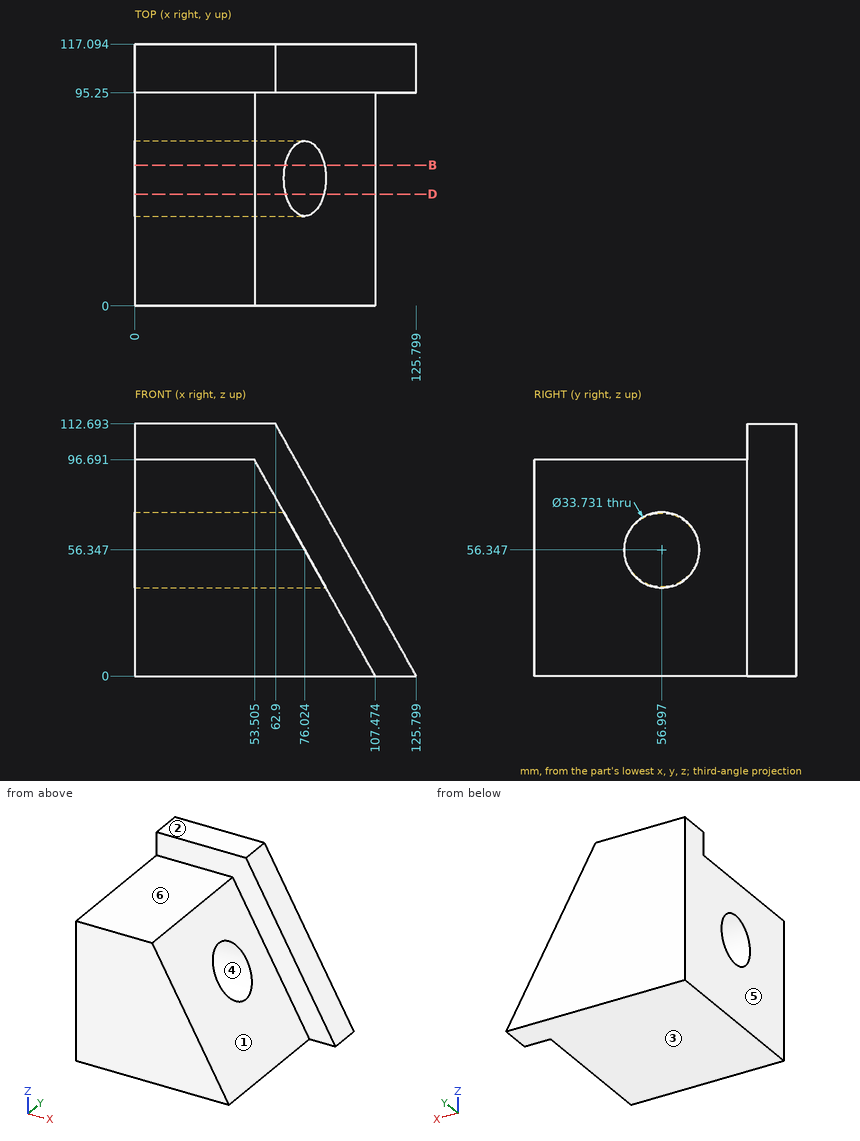
Part print with two shaded views. Sizes in mm from the minimum x, y, z corner. A direction names the side the tool comes from. Give positions to 0.01 mm unless a question says otherwise; leave off trailing zeros. Order: outer loops, then holes, each group sorted by start corner. A loop starts at its lowest first (then second) coordinate and runs counter-clockwise, first axis right, second up. Notation, with made-up numbers: (8, 78) - (66, 78) arc R19 ccw to (66, 104) - close; hole circle Ø2 at (9, 11.5). An arc over 180 degrees is marked (long way). Write each question's results on one line, items separated by ' | '.
1. Pull direction Z, two halves, no side cores. Call the marked faces 3, 4, 5 and 6: released by +Z, released by -Z, zero draft, split by the parting line, or undercut.
Calculated:
face 3: released by -Z | face 4: undercut | face 5: zero draft | face 6: released by +Z
2. 3-axis set-ups, long thin cutter, end or side, ignore diameter. For the marked faces 1 and 2: which of +Z, -Z, +X, -X, +Y, -Y reach the whole face in a straight line?
Calculated:
face 1: +Z, +X, -Y | face 2: +Z, +X, -X, +Y, -Y
3. Saw through at B-B on y = 63. List the corners of the cut face in (x, z) (1 decimal).
Calculated:
outline: (0, 0) - (107.5, 0) - (84.8, 40.6) - (0, 40.6) - close; (0, 72.1) - (67.2, 72.1) - (53.5, 96.7) - (0, 96.7) - close
4. Probe L1, parallel to Y at x = 79, z = 67.5; L2, parallel to Y at x = 26.5, z = 51 (1 decimal); L3, parallel to Z at x = 11, y = 61. List the from-to ranges inside material, lowest first. Write a range as from..to.
Calculated:
L1: y = 95.25..117.09 | L2: y = 0..41, 73..117.1 | L3: z = 0..39.96, 72.73..96.69
5. Pin check, flat tips, straight feed: pin 1 (4 mm diameter, centred on x = 32, y = 24, fed in from +Z); pin 2 (5 mm diameter, centred on x = 29.5, z = 64, fed in from -Y); pin 3 (12 mm diameter, centred on x = 77.5, z = 74, fed in from -Y); pin 4 (10 mm diameter, centred on y = 98, z = 38, fed in from +X). Stop position of each tip, or through.
Calculated:
pin 1: stops at z = 96.69 | pin 2: stops at y = 0 | pin 3: stops at y = 95.25 | pin 4: stops at x = 107.38
6. Saw through at D-D on y = 50. List the corners of the cut face in (x, z) (1 decimal), and give its area (3 significant figures).
Calculated:
outline: (0, 0) - (107.5, 0) - (84.6, 41) - (0, 41) - close; (0, 71.7) - (67.5, 71.7) - (53.5, 96.7) - (0, 96.7) - close | area: 5,450 mm2
